from build123d import *

# Parameters (mm, degrees)
SKETCH1_W            = 59.999999999
SKETCH1_H            = 32
BOSS_EXTRUDE1_DEPTH  = 25.1
M5_CLEARANCE_HOLE1_D = 5.4
FILLET1_R            = 3
BOSS_EXTRUDE2_DEPTH  = 25.1


with BuildPart() as part:
    # Sketch1 → Boss-Extrude1 (new body)
    with BuildSketch(Plane.XY):
        with Locations((8.905545777, 63)):
            Rectangle(SKETCH1_W, SKETCH1_H)
    extrude(amount=BOSS_EXTRUDE1_DEPTH)

    # M5 Clearance Hole1 (through all)
    with Locations(Plane(origin=(0, 0, 25.1), x_dir=(-1, 0, 0), z_dir=(0, 0, 1))):
        with Locations((-31.905545776, -72), (-31.905545776, -54), (14.094454224, -54), (14.094454224, -72)):
            Hole(M5_CLEARANCE_HOLE1_D / 2)

    # Fillet1
    fillet1_edges = [part.edges().sort_by_distance(p)[0] for p in [
        (-21.094454223, 47, 12.55),
        (-21.094454223, 79, 12.55),
        (38.905545776, 79, 12.55),
        (38.905545776, 47, 12.55),
    ]]
    fillet(fillet1_edges, radius=FILLET1_R)

    # Sketch4 → Boss-Extrude2 (add)
    with BuildSketch(Plane.XY.offset(25.1)):
        with BuildLine():
            Line((42.905545776, 50), (42.905545776, 76))
            ThreePointArc((42.905545776, 76), (40.855293244, 80.949747468), (35.905545776, 83))
            Line((35.905545776, 83), (-18.094454223, 83))
            ThreePointArc((-18.094454223, 83), (-23.044201691, 80.949747468), (-25.094454223, 76))
            Line((-25.094454223, 76), (-25.094454223, 50))
            ThreePointArc((-25.094454223, 50), (-23.044201691, 45.050252532), (-18.094454223, 43))
            Line((-18.094454223, 43), (35.905545776, 43))
            ThreePointArc((35.905545776, 43), (40.855293244, 45.050252532), (42.905545776, 50))
        make_face()
        with BuildLine():
            Line((35.905545776, 79), (-18.094454223, 79))
            ThreePointArc((-18.094454223, 79), (-20.215774567, 78.121320343), (-21.094454223, 76))
            Line((-21.094454223, 76), (-21.094454223, 50))
            ThreePointArc((-21.094454223, 50), (-20.215774567, 47.878679656), (-18.094454223, 47))
            Line((-18.094454223, 47), (35.905545776, 47))
            ThreePointArc((35.905545776, 47), (38.026866119, 47.878679656), (38.905545776, 50))
            Line((38.905545776, 50), (38.905545776, 76))
            ThreePointArc((38.905545776, 76), (38.026866119, 78.121320343), (35.905545776, 79))
        make_face(mode=Mode.SUBTRACT)
    extrude(amount=-BOSS_EXTRUDE2_DEPTH)


solid = part.part
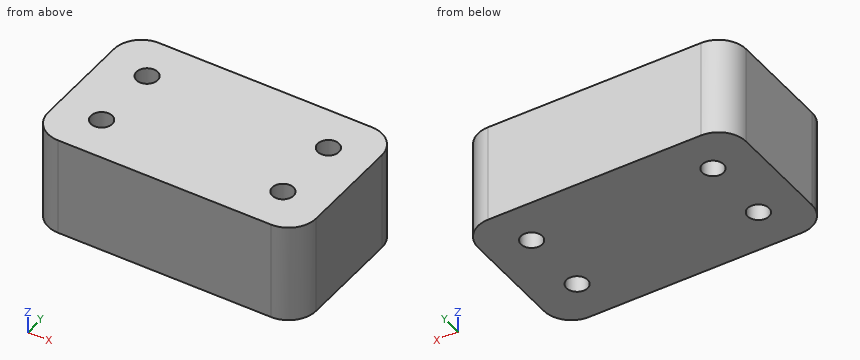
Check sheet for the modelled part. Datum: model origin and axes. Units: mm. Round coordinates to 2 decimals unless told otherwise and drop trailing zeros. Order: outer loops, then holes, each group sorted by start corner. A loop starts at its lowest first (then second) coordinate and runs counter-clockwise, first axis right, second up. Notation, with made-up numbers: M -7,84 L 0,84 A15 ccw 0,92 Z; hole C 15,15 d4. An arc over 180 degrees is marked long. One line per item, written item: value. Start each with the question number.
1. Section check A-A on y = 72. Enter the section's corners in (x, z), and give its area (3 significant figures).
2. Section check C-C on x = -14.5. Enter the section's corners in (y, z), and give its area (3 significant figures).
3. Section check D-D on y = 79. Enter the section's corners in (x, z).
4. Scan lines: line 1 along X through (y, z) = (72, 15.5); line 2 along Y through (x, z) = (-15, 8); line 3 along X through (y, z) = (54.5, 22.75). Record each from-to range of solid material in increasing order.
5. Section check B-B on z = 22.5. Enter the section's corners in (x, y), and give its area (3 significant figures).
Results found:
1. outline: M -25.09,0 L -16.79,0 L -16.79,25.1 L -25.09,25.1 Z; M -11.39,0 L 29.21,0 L 29.21,25.1 L -11.39,25.1 Z; M 34.61,0 L 42.91,0 L 42.91,25.1 L 34.61,25.1 Z
1. area: 1,440 mm^2
2. outline: M 43,0 L 51.33,0 L 51.33,25.1 L 43,25.1 Z; M 56.67,0 L 69.33,0 L 69.33,25.1 L 56.67,25.1 Z; M 74.67,0 L 83,0 L 83,25.1 L 74.67,25.1 Z
2. area: 736 mm^2
3. outline: M -24.42,0 L 42.23,0 L 42.23,25.1 L -24.42,25.1 Z
4. line 1: -25.09 to -16.79, -11.39 to 29.21, 34.61 to 42.91
4. line 2: 43 to 51.46, 56.54 to 69.46, 74.54 to 83
4. line 3: -25.09 to -16.75, -11.44 to 29.25, 34.56 to 42.91
5. outline: M -25.09,50 A7 ccw -18.09,43 L 35.91,43 A7 ccw 42.91,50 L 42.91,76 A7 ccw 35.91,83 L -18.09,83 A7 ccw -25.09,76 Z; hole C -14.09,54 d5.4; hole C -14.09,72 d5.4; hole C 31.91,54 d5.4; hole C 31.91,72 d5.4
5. area: 2,590 mm^2
